Work out the finished part from the listing and answer in its coordinate system (mm). Coordinates: 2 decimals unless noted, no trailing zeros. Order: outer loops, then holes, each group sorted by start corner. A loop starts at its lowest first (then second) coordinate and runs counter-clockwise, first axis right, second up. Notation, with made-up numbers: (24, 29.5) -> (37, 29.5) arc R28 cw to (37, 59.5) -> close; hole circle Ø8 at (74.25, 31.25). An arc over 180 degrees is marked (long way). Write item = value, one per line. Start each with the question number.
Q1. Flat-ended cylindrical pins translate along their axes: pin 1 (6.5 mm diameter, centred on x = -2, z = -3, fed in from +Y); pin 2 (3 mm diameter, centred on y = 2, z = 27, fed in from -X); pin 3 (3 mm diameter, centred on x = 42.5, y = 5.5, fed in from +Z). Find the tip coordinate at first contact, or state that the pin passes through.
Q2. The part is cut by section B-B, the plane y = 3.25. Determine the outline of the cut face in (x, z).
Q3. The part is cut by section C-C, the plane z = -46.5. Determine the outline of the cut face in (x, y), plus the area to 3 significant figures.
Q4. The part is cut by section A-A, the plane z = 0. Determine the outline of the cut face in (x, y).
Q5. Straight lines are drawn through the part: L1, parallel to X at y = 0.25, z = 0; L2, parallel to Z at x = 1.5, y = 3.4; L3, parallel to X at y = 4.55, z = 29.5. For each, find the intervals that lie inside material, in ascending order. Write a range as from..to.
Q6. The part is cut by section D-D, the plane x = -36.5. Determine the outline of the cut face in (y, z), plus the area to 3 significant figures.
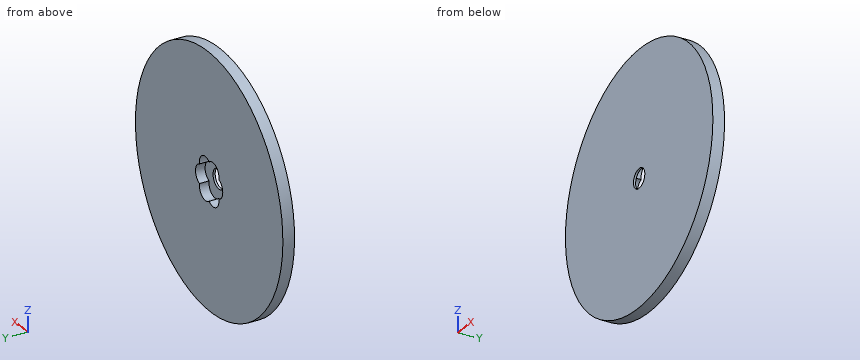
```python
from build123d import *

# Parameters (mm, degrees)
SKETCH1_R           = 65
BOSS_EXTRUDE1_DEPTH = 6
SKETCH2_R           = 5
CUT_EXTRUDE1_DEPTH  = 93.119487623
SKETCH3_R           = 5.243686523
CUT_EXTRUDE2_DEPTH  = 4.901436
CIRPATTERN1_START   = 1.09856408
CIRPATTERN1_DEPTH   = 4.90143592


# Read off the part's stored shape, not the designer's step: CirPattern1
with BuildPart() as part:
    # Sketch1 → Boss-Extrude1 (new body)
    with BuildSketch(Plane(origin=(0, 0, 0), x_dir=(1, 0, 0), z_dir=(0, 1, 0))):
        with Locations(Location((0, 0, 0), (0, 0, 270))):
            Circle(SKETCH1_R)
    extrude(amount=BOSS_EXTRUDE1_DEPTH)

    # Sketch2 → Cut-Extrude1 (cut, through all)
    with BuildSketch(Plane(origin=(0, 0, 0), x_dir=(1, 0, 0), z_dir=(0, 1, 0))):
        with Locations(Location((0, 0, 0), (0, 0, 270))):
            Circle(SKETCH2_R)
    extrude(amount=CUT_EXTRUDE1_DEPTH, mode=Mode.SUBTRACT)

    # Sketch3 → Cut-Extrude2 (cut)
    with BuildSketch(Plane(origin=(0, 6, 0), x_dir=(1, 0, 0), z_dir=(0, 1, 0))):
        with Locations((-6.759613597, 0)):
            Circle(SKETCH3_R)
    extrude(amount=-CUT_EXTRUDE2_DEPTH, mode=Mode.SUBTRACT)

    # CirPattern1 outline → CirPattern1 (cut)
    with BuildSketch(Plane(origin=(0, 0, 0), x_dir=(1, 0, 0), z_dir=(0, 1, 0)).offset(CIRPATTERN1_START)):
        with BuildLine():
            ThreePointArc((-3.19516249, -3.845898681), (-5.716131684, -5.138812495), (-8.541721973, -4.931565481))
            ThreePointArc((-8.541721973, -4.931565481), (-6.00165006, -10.395162834), (0, -9.863130961))
            ThreePointArc((0, -9.863130961), (6.00165006, -10.395162834), (8.541721973, -4.931565481))
            ThreePointArc((8.541721973, -4.931565481), (12.00330012, 0), (8.541721973, 4.931565481))
            ThreePointArc((8.541721973, 4.931565481), (6.00165006, 10.395162834), (0, 9.863130961))
            ThreePointArc((0, 9.863130961), (-6.00165006, 10.395162834), (-8.541721973, 4.931565481))
            ThreePointArc((-8.541721973, 4.931565481), (-5.716131684, 5.138812495), (-3.19516249, 3.845898681))
            ThreePointArc((-3.19516249, 3.845898681), (5, 0), (-3.19516249, -3.845898681))
        make_face()
    extrude(amount=CIRPATTERN1_DEPTH, mode=Mode.SUBTRACT)


solid = part.part
```
Model answer:
q1.pin_1 = 1.1
q1.pin_2 = -59.79
q1.pin_3 = 50.44
q2.outline = circle Ø130 at (0, 0); hole (-8.54, -4.93) arc R5.24 ccw to (0, -9.86) arc R5.24 ccw to (8.54, -4.93) arc R5.24 ccw to (8.54, 4.93) arc R5.24 ccw to (0, 9.86) arc R5.24 ccw to (-8.54, 4.93) arc R5.24 ccw to start
q3.outline = (-45.42, 0) -> (45.42, 0) -> (45.42, 6) -> (-45.42, 6) -> close
q3.area = 545 mm2
q4.outline = (-65, 0) -> (-5, 0) -> (-5, 1.1) -> (-12, 1.1) -> (-12, 6) -> (-65, 6) -> close; (5, 0) -> (65, 0) -> (65, 6) -> (12, 6) -> (12, 1.1) -> (5, 1.1) -> close
q5.L1 = -65..-5, 5..65
q5.L2 = -64.98..-10.75, 10.75..64.98
q5.L3 = -57.92..57.92
q6.outline = (0, -53.78) -> (6, -53.78) -> (6, 53.78) -> (0, 53.78) -> close
q6.area = 645 mm2
